Input: part model. Units: mm. Frame: model coordinates. Face numbers are marked on the shaded views. Round coordinates to 2 decimals unless told otherwise and drop trailing zeros. Loops run counter-clockwise (first coordinate to the right, second up) from the corner with the lowest first, then second, coordinate; pieces in that order, holes last. Notation, with made-up numbers: (-9.75, 34.5) -> (21.25, 34.5) arc R26 ccw to (21.25, 63.5) -> close; hole circle Ø8 at (85.25, -32). An arc over 180 degrees is marked (long way). One line per question, with ' | ' between items. Start each with the question number.
Q1. Cut plane C-C on z = 4. Return loops of the section in (x, y).
Q2. Contact query for a flat-ended pin moving along its axis: P1, Ø6, axis at x = -1.5, z = 5, coming from the -Y side. Output: stop coordinate, or through.
Q3. Cut plane A-A on x = 0. Return loops of the section in (y, z).
Q4. Material intervals for L1, parallel to Z at x = 0, y = -1.75; L2, parallel to X at y = -3, z = 4; L3, parallel to X at y = -2.25, z = 4, sorted ascending.
Q5. Mould query, pull axis X, two halves, no side actions, for the marked faces 1, 2 and 3. Classes: pulls with the +X half, pulls with the -X half, needs draft (parallel to the pull), parting line crosses it, or undercut.
Q6. Cut plane B-B on y = -6.5. Return loops of the section in (x, z).
Q7. Cut plane D-D on y = -2.75. Return loops of the section in (x, z).
Autodesk Inventor part; units mm, degrees
ref_plane "MidPlane" through (-6.9, 0, 0) normal (0, 0, -1) x (-1, 0, 0)
ref_plane "Work Plane4" through (6.9, 0, -3.8333) normal (0, 0, -1) x (-1, 0, 0)
ref_plane "YZ Plane" through (0, 0, 0) normal (1, 0, 0) x (0, 1, 0)
sketch "Sketch2" plane through (0, 0, 0) normal (0, 1, 0) x (-1, 0, 0)
  line L0 (6.9, -11.5) -> (-6.9, -11.5)
  line L1 (-6.9, -11.5) -> (-6.9, 11.5)
  line L2 (-6.9, 11.5) -> (6.9, 11.5)
  line L3 (6.9, 11.5) -> (6.9, -11.5)
  point P0 (0, 4)
  point P1 (0, -11.5)
  point P2 (0, 11.5)
  point P3 (0, 0)
  point P4 (-6.9, 0)
  dimension "CenterHole" = 7.5
  dimension "Length" = 23
  dimension "Width" = 13.8
extrude "NutBase" add sketch "Sketch2" against normal blind 7.3
hole "Hole1" at (0, 0, 4) direction (0, -1, 0) diameter 6.647 end through all
ref_plane "MidPlane" through (-6.9, 0, 0) normal (0, 0, -1) x (-1, 0, 0)
ref_plane "Work Plane4" through (6.9, 0, -3.8333) normal (0, 0, -1) x (-1, 0, 0)
sketch "Sketch3" plane through (-6.9, 0, 11.5) normal (0, 0, 1) x (1, 0, 0)
  line L0 (0, -7.3) -> (13.8, -7.3) construction
  line L1 (13.8, 0) -> (0, 0)
  line L2 (0, 0) -> (2.3, -4.4884)
  arc A0 (2.3, -4.4884) -> (11.5, -4.4884) centre (6.9, -2.1312) ccw
  line L3 (11.5, -4.4884) -> (13.8, 0)
  line L4 (6.9, -2.1312) -> (6.9, 0) construction
  dimension "d12" = 9.2
extrude "Standard TSlot" cut sketch "Sketch3" along normal through all both and the other way through all keep common part
sketch "Sketch5" plane through (-6.9, 0, 11.5) normal (0, 0, 1) x (1, 0, 0)
  line L0 (0, -7.3) -> (13.8, -7.3) construction
  line L1 (13.8, 0) -> (0, 0)
  line L2 (0, 0) -> (0, -7.3) construction
  line L3 (6.9, 0) -> (6.9, -7.3) construction
  line L4 (0, -0.8) -> (2.95, -0.8)
  line L5 (2.95, -0.8) -> (2.95, 0)
  line L6 (2.95, 0) -> (0, 0)
  line L7 (0, 0) -> (0, -0.8)
  line L8 (13.8, -0.8) -> (10.85, -0.8)
  line L9 (10.85, -0.8) -> (10.85, 0)
  line L10 (10.85, 0) -> (13.8, 0)
  line L11 (13.8, 0) -> (13.8, -0.8)
  dimension "Slot_Width" = 7.9
  dimension "d18" = 0.8
extrude "Self-Align TSlot" [suppressed]
sketch "Sketch6" plane through (-6.9, 0, 11.5) normal (0, 0, 1) x (1, 0, 0)
  line L0 (0, -7.3) -> (13.8, -7.3)
  line L1 (13.8, 0) -> (13.8, -7.3)
  line L2 (13.8, 0) -> (0, 0)
  line L3 (0, 0) -> (0, -7.3)
  line L4 (6.9, 0) -> (6.9, -7.3) construction
  line L5 (0, 0) -> (2.95, 0)
  line L6 (2.95, 0) -> (2.95, -3.5)
  line L7 (2.95, -3.5) -> (0, -3.5)
  line L8 (0, -3.5) -> (0, 0)
  line L9 (13.8, 0) -> (10.85, 0)
  line L10 (10.85, 0) -> (10.85, -3.5)
  line L11 (10.85, -3.5) -> (13.8, -3.5)
  line L12 (13.8, -3.5) -> (13.8, 0)
  arc A0 (0, -4.8) -> (2.5, -7.3) centre (2.5, -4.8) ccw
  arc A1 (11.3, -7.3) -> (13.8, -4.8) centre (11.3, -4.8) ccw
  dimension "HD_Slot_Depth" = 3.5
  dimension "HD_Slot_Width" = 7.9
  dimension "d23" = 2.5
extrude "Heavy Duty TSlot" [suppressed]
sketch "Sketch7" plane through (0, 0, 0) normal (0, 1, 0) x (1, 0, 0)
  line L0 (-6.9, 11.5) -> (6.9, 11.5)
  line L1 (-6.9, -11.5) -> (-6.9, 11.5)
  line L2 (6.9, -11.5) -> (-6.9, -11.5)
  line L3 (6.9, 11.5) -> (6.9, -11.5)
  arc A0 (6.9, 8.7381) -> (-6.9, 8.7381) centre (0, 1.5) ccw
  arc A1 (-6.9, -8.7381) -> (6.9, -8.7381) centre (0, -1.5) ccw
  line L4 (-9.66, 0) -> (9.66, 0) construction
  point P0 (0, 11.5)
  point P1 (0, -11.5)
  dimension "Economy_Fillet_Size" = 10
extrude "Economy TSlot" [suppressed]
sketch "Sketch9" plane through (0, -7.3, 0) normal (0, -1, 0) x (1, 0, 0)
  arc A0 (8, 8.5) -> (-8, 8.5) centre (0, 2.5) ccw
  line L0 (-9.5459, -8.5) -> (-9.5459, 8.5)
  arc A1 (-8, -8.5) -> (8, -8.5) centre (0, -2.5) ccw
  line L1 (9.5459, 8.5) -> (9.5459, -8.5)
  circle A2 centre (0, 4) radius 3.3235 construction
  circle A3 centre (0, 4) radius 4.5735
  dimension "d35" = 1.25
extrude "Economy TSlot2" [suppressed]
sketch "Sketch4" plane through (6.9, 0, -3.8333) normal (0, 0, -1) x (-1, 0, 0)
  circle A0 centre (6.9, -7.05) radius 0.75
  line L0 (6.9276, -6.3005) -> (6.8724, -6.3005)
  line L1 (6.9, -9.36) -> (6.9, 1.56) construction
  line L2 (13.8, -7.3) -> (0, -7.3) construction
  line L3 (6.9, -6.3005) -> (6.9, -7.8)
  line L4 (0, 0) -> (13.8, 0) construction
  dimension "d15" = 1.5
  dimension "d38" = 7.05
revolve "SpringBall" add sketch "Sketch4" angle 360 about axis through (0, -10, -3.8333) along (0, 1, 0) picked at (6.8409, -7.2931) contours A0 L3
mirror "Double Mirror" [suppressed]
sketch "Sketch10" plane through (-6.9, 0, 11.5) normal (0, 0, 1) x (1, 0, 0)
  line L0 (6.9, -8.76) -> (6.9, 1.46) construction
  line L1 (0, 0) -> (4.0362, 0)
  line L2 (4.0362, 0) -> (4.0362, -1.925)
  line L3 (4.0362, -1.925) -> (0, -1.925)
  line L4 (0, -1.925) -> (0, 0)
  line L5 (13.8, 0) -> (9.7638, 0)
  line L6 (9.7638, 0) -> (9.7638, -1.925)
  line L7 (9.7638, -1.925) -> (13.8, -1.925)
  line L8 (13.8, -1.925) -> (13.8, 0)
  dimension "d40" = 5.7276
  dimension "d41" = 1.925
extrude "Zn TSlot 1" [suppressed]
sketch "Sketch11" plane through (0, -7.3, 0) normal (0, -1, 0) x (1, 0, 0)
  circle A0 centre (0, 4) radius 3.3235
  line L0 (-6.9, -11.5) -> (-6.9, 11.5)
  line L1 (6.9, -11.5) -> (-6.9, -11.5)
  line L2 (6.9, -11.5) -> (-6.9, 2.3)
  line L3 (0, 4) -> (-6.9, 10.9) construction
  line L4 (6.9, 11.5) -> (6.9, -11.5)
  line L5 (-6.9, 11.5) -> (6.9, -2.3)
  line L6 (-6.9, 11.5) -> (6.9, 11.5)
  dimension "d44" = 45
  dimension "d45" = 12.1622
  dimension "d48" = 45
extrude "Zn TSlot 2" [suppressed]
equation "\"d12\" = 0.666667 * Width"
equation "\"HD_Slot_Width\" = Slot_Width"
equation "\"d40\" = 0.707107 * Zn_C"
equation "\"d41\" = 0.25 * Zn_E"
equation "\"SpringBallPos\" = -0.333333 * Length"
equation "\"Zn_B\" = 27"
equation "\"Zn_C\" = 8.1"
equation "\"Zn_D\" = 7.9"
equation "\"Zn_E\" = 7.7"
properties part number "20-058" material "Steel, High Strength Low Alloy"
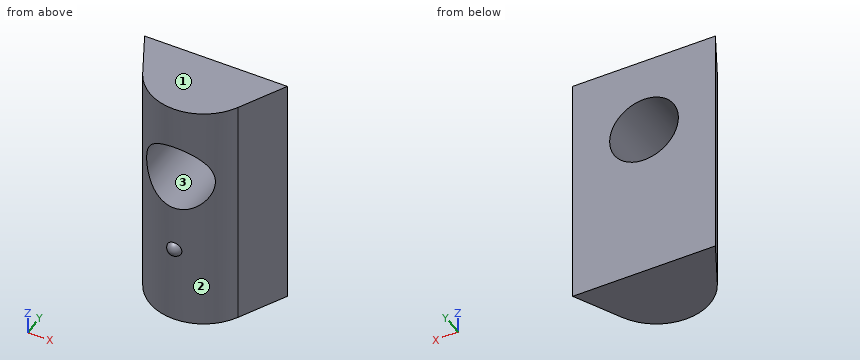
Results:
1) outline: (-6.9, 0) -> (-4.6, -4.49) arc R5.17 ccw to (-3.32, -6.09) -> (-3.32, 0) -> close; (3.32, -6.09) arc R5.17 ccw to (4.6, -4.49) -> (6.9, 0) -> (3.32, 0) -> close
2) P1: y = -7.3
3) outline: (-7.3, -11.5) -> (0, -11.5) -> (0, 0.68) -> (-7.3, 0.68) -> (-7.3, -3.13) arc R0.75 ccw to (-7.3, -4.54) -> close; (-7.3, 7.32) -> (0, 7.32) -> (0, 11.5) -> (-7.3, 11.5) -> close
4) L1: -11.5 to 0.68, 7.32 to 11.5 | L2: -5.36 to -3.32, 3.32 to 5.36 | L3: -5.75 to -3.32, 3.32 to 5.75
5) face 1: needs draft | face 2: parting line crosses it | face 3: undercut
6) outline: (-2.76, -11.5) -> (2.76, -11.5) -> (2.76, 2.15) arc R3.32 cw to (-2.76, 2.15) -> close; (-2.76, 5.85) arc R3.32 cw to (2.76, 5.85) -> (2.76, 11.5) -> (-2.76, 11.5) -> close
7) outline: (-5.49, -11.5) -> (5.49, -11.5) -> (5.49, 11.5) -> (-5.49, 11.5) -> close; hole circle Ø6.65 at (0, 4)
